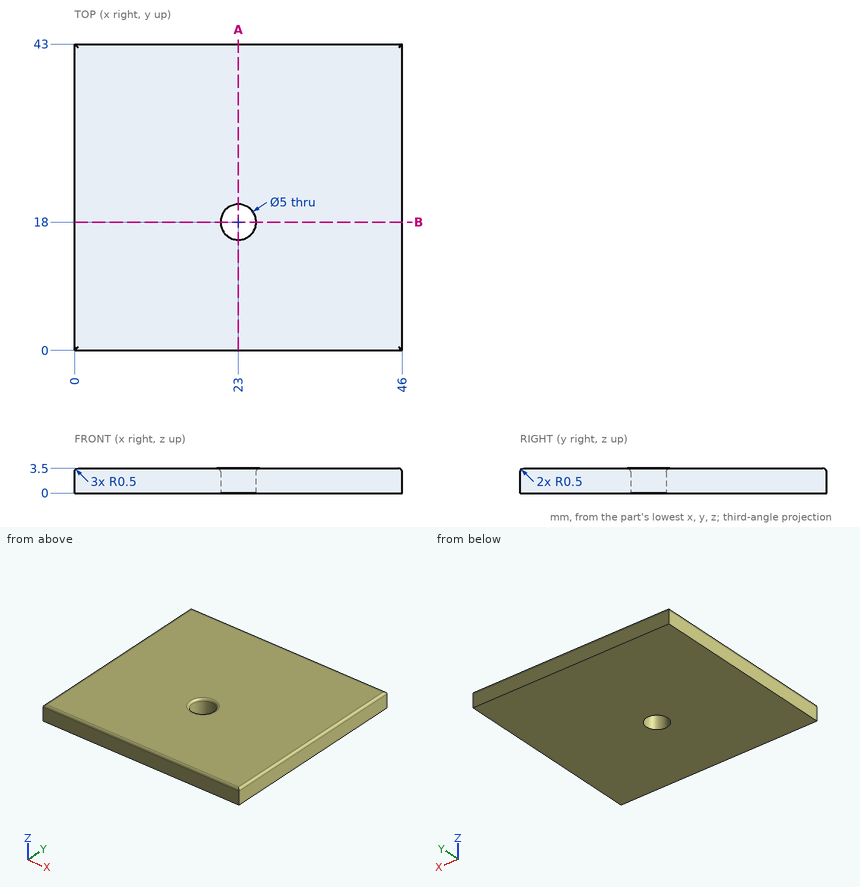
The drawing under review shows one solid part. Ordinate dimensions are in mm from its lowest x, y, z. Give positions to 0.01 mm unless a question says otherwise; leave off trailing zeros. Order: outer loops, then holes, each group sorted by start corner. A loop starts at its lowest first (then second) coordinate and runs counter-clockwise, first axis right, second up. Notation, with made-up numbers: (-22, 87) - (24, 87) arc R12 cw to (24, 94) - close; hole circle Ø2 at (-12.5, 65.5). An arc over 180 degrees is marked (long way). Answer as a JSON object with one key per item and string values. Group by question number.
Item 1: Wall thickness on line 1 along Y through (x, z) = (23, 1.45); line 2 along X through (y, z) = (19, 1.3); line 3 along X through (y, z) = (38.5, 3.25): over which ranges is each line inside the solid? List them lowest first.
Item 2: Take a section at A-A on x = 23. Give the boundary of the cut face in (y, z), and give its area (3 significant figures).
Item 3: Take a section at B-B on y = 18. Give the boundary of the cut face in (x, z), and give its area (3 significant figures).
Item 4: Clearance check with flat-ended pins moving along their axes: pin 1 Ø4 at (x, y) = (23, 18) entering from -Z (3 decimals); pin 2 Ø1 at (y, z) = (28, 2.5) entering from -X. State where each tip first meets the part, or that it passes through.
Reported:
{
 "1": {"line 1": "0 to 15.5, 20.5 to 43", "line 2": "0 to 20.71, 25.29 to 46", "line 3": "0.07 to 45.93"},
 "2": {"outline": "(0, 0) - (15.5, 0) - (15.5, 3) arc R0.5 ccw to (15, 3.5) - (0.5, 3.5) arc R0.5 ccw to (0, 3) - close; (20.5, 0) - (43, 0) - (43, 3) arc R0.5 ccw to (42.5, 3.5) - (21, 3.5) arc R0.5 ccw to (20.5, 3) - close", "area": "133 mm^2"},
 "3": {"outline": "(0, 0) - (20.5, 0) - (20.5, 3) arc R0.5 ccw to (20, 3.5) - (0.5, 3.5) arc R0.5 ccw to (0, 3) - close; (25.5, 0) - (46, 0) - (46, 3) arc R0.5 ccw to (45.5, 3.5) - (26, 3.5) arc R0.5 ccw to (25.5, 3) - close", "area": "143 mm^2"},
 "4": {"pin 1": "through", "pin 2": "x = 0"}
}
